Input: part model. Units: mm. Frame: model coordinates. Face numbers are marked on the shaded views. A direction names the side the tool comes from. Coordinates: 2 decimals unless noted, no trailing zeros. Loops run counter-clockwise (first coordinate to the right, second up) from the corner with the lowest first, then second, coordinate; pieces in that order, holes last.
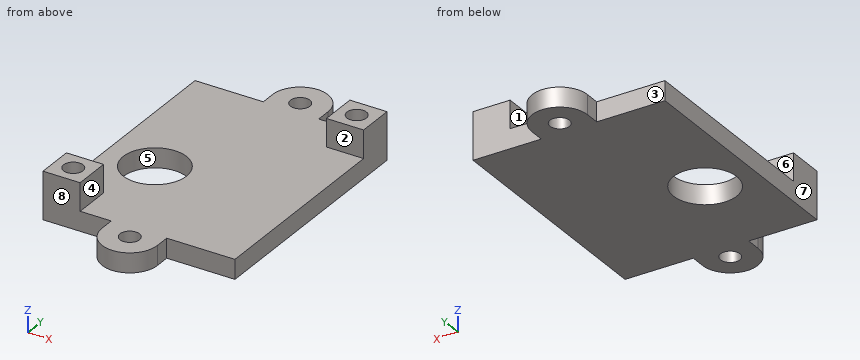
```python
from build123d import *

# Parameters (mm, degrees)
PAD_DEPTH       = 4
SKETCH001_R     = 6.5
POCKET_DEPTH    = 5
SKETCH002_W     = 7.62
SKETCH002_H     = 7.62
PAD001_DEPTH    = 5.7
SKETCH003_R     = 2
POCKET001_DEPTH = 5.7
SKETCH004_R     = 2
POCKET002_DEPTH = 5


with BuildPart() as part:
    # Sketch → Pad (new body)
    with BuildSketch(Plane.XY):
        with BuildLine():
            Line((0, 0), (0, 49.53))
            Line((0, 49.53), (14, 49.53))
            Line((14, 49.53), (14, 52.53))
            ThreePointArc((25.37, 52.53), (19.685, 58.215), (14, 52.53))
            Line((25.37, 49.53), (25.37, 52.53))
            Line((25.37, 49.53), (39.37, 49.53))
            Line((39.37, 49.53), (39.37, 0))
            Line((39.37, 0), (25.37, 0))
            Line((25.37, 0), (25.37, -3))
            ThreePointArc((14, -3), (19.685, -8.685027), (25.37, -3))
            Line((14, 0), (14, -3))
            Line((0, 0), (14, 0))
        make_face()
    extrude(amount=PAD_DEPTH)

    # Sketch001 (on Face14 of Pad) → Pocket (cut)
    with BuildSketch(Plane.XY.offset(4)):
        with Locations((10.16, 20.31)):
            Circle(SKETCH001_R)
    extrude(amount=-POCKET_DEPTH, mode=Mode.SUBTRACT)

    # Sketch002 (on Face5 of Pocket) → Pad001 (join)
    with BuildSketch(Plane.XY.offset(4)):
        with Locations((3.81, 3.81)):
            Rectangle(SKETCH002_W, SKETCH002_H)
        with Locations((35.56, 45.72)):
            Rectangle(SKETCH002_W, SKETCH002_H)
    extrude(amount=PAD001_DEPTH)

    # Sketch003 (on Face19 of Pad001) → Pocket001 (cut)
    with BuildSketch(Plane.XY.offset(9.7)):
        with Locations((3.81, 3.81)):
            Circle(SKETCH003_R)
        with Locations((35.56, 45.72)):
            Circle(SKETCH003_R)
    extrude(amount=-POCKET001_DEPTH, mode=Mode.SUBTRACT)

    # Sketch004 (on Face6 of Pocket001) → Pocket002 (cut)
    with BuildSketch(Plane.XY.offset(4)):
        with Locations((19.685, -3.000027)):
            Circle(SKETCH004_R)
        with Locations((19.685, 52.53)):
            Circle(SKETCH004_R)
    extrude(amount=-POCKET002_DEPTH, mode=Mode.SUBTRACT)


solid = part.part
```
Item 1: Reachability of the marked faces 1, 2, 3 and 4 from +Z, -Z, +X, -X, +Y, -Y: full face, straight path, thin tool, end or side. Return the list, or none.
Result:
face 1: +Z, -X, +Y, -Y
face 2: +Z, +X, -X, -Y
face 3: +Z, -Z, -X, +Y
face 4: +Z, +X, +Y, -Y
Item 2: Mould query, pull axis Y, two halves, no side actions, for the marked faces 5, 6, 7 and 8. Classes: +Y half, -Y half, draft (parallel to the pull), parting line (faces both ways), or undercut.
Result:
face 5: undercut
face 6: +Y half
face 7: draft
face 8: -Y half
Item 3: Section query D-D (z = 1.75). Output: boundary loops of the cut face in (x, y) (3 decimals).
Result:
outline: (0, 0) - (14, 0) - (14, -3) arc R5.685 ccw to (25.37, -3) - (25.37, 0) - (39.37, 0) - (39.37, 49.53) - (25.37, 49.53) - (25.37, 52.53) arc R5.685 ccw to (14, 52.53) - (14, 49.53) - (0, 49.53) - close; hole circle Ø13 at (10.16, 20.31); hole circle Ø4 at (19.685, -3); hole circle Ø4 at (19.685, 52.53)
Item 4: Section query B-B (x = 10.16). Output: boundary loops of the cut face in (y, z).
Result:
outline: (0, 0) - (13.81, 0) - (13.81, 4) - (0, 4) - close; (26.81, 0) - (49.53, 0) - (49.53, 4) - (26.81, 4) - close
Item 5: Section query A-A (z = 5). Output: boundary loops of the cut face in (x, y).
Result:
outline: (0, 0) - (7.62, 0) - (7.62, 7.62) - (0, 7.62) - close; (31.75, 41.91) - (39.37, 41.91) - (39.37, 49.53) - (31.75, 49.53) - close; hole circle Ø4 at (3.81, 3.81); hole circle Ø4 at (35.56, 45.72)
Item 6: Contact query for flat-ended pins moving along their axis: P1, Ø1.5, axis at y = 50.5, z = 2.5, coming from the +X side; P2, Ø1.2, axis at x = 29, z = 2.5, coming from the -Y side; P3, Ø1.2, axis at x = 7, z = 1.5, coming from the +Y side; P4, Ø2.5, axis at x = 19.68, y = -3, coming from the -Z side. Output: stop coordinate, or through.
Result:
P1: stops at x = 25.37
P2: stops at y = 0
P3: stops at y = 49.53
P4: passes through
Item 7: Section query C-C (x = 35.56). Output: boundary loops of the cut face in (y, z), then the cut area to 3 significant figures.
Result:
outline: (0, 0) - (49.53, 0) - (49.53, 9.7) - (47.72, 9.7) - (47.72, 4) - (43.72, 4) - (43.72, 9.7) - (41.91, 9.7) - (41.91, 4) - (0, 4) - close
area: 219 mm2
Item 8: Line query: L1, parallel to Y at x = 4, z = 5.25; L2, parallel to Z at x = 14.5, y = 1; L3, parallel to Y at x = 35.56, z = 5.35. Output: solid intervals per line, ascending.
Result:
L1: y = 0 to 1.82, 5.8 to 7.62
L2: z = 0 to 4
L3: y = 41.91 to 43.72, 47.72 to 49.53
